```python
from build123d import *

# Parameters (mm, degrees)
ESQUISSE1_R             = 6
ESQUISSE1_R_2           = 1.6
EXTRUSION1_DEPTH        = 5
ESQUISSE2_W             = 10
ESQUISSE2_H             = 6
ENL_V_MAT_EXTRU_1_DEPTH = 2.5
ESQUISSE3_R             = 1.5
ENL_V_MAT_EXTRU_2_DEPTH = 28.658633372


with BuildPart() as part:
    # Esquisse1 → Extrusion1 (new body)
    with BuildSketch(Plane.XY):
        Polygon((-7, 16), (10, 16), (10, -16), (-7, -16), (-7, -7.5), (-12, -7.5), (-12, 7.5), (-7, 7.5), align=None)
        Circle(ESQUISSE1_R, mode=Mode.SUBTRACT)
        with Locations((-9, 0)):
            Circle(ESQUISSE1_R_2, mode=Mode.SUBTRACT)
        with Locations((4.5, 7.794228634)):
            Circle(ESQUISSE1_R_2, mode=Mode.SUBTRACT)
        with Locations((4.5, -7.794228634)):
            Circle(ESQUISSE1_R_2, mode=Mode.SUBTRACT)
    extrude(amount=EXTRUSION1_DEPTH)

    # Esquisse2 → Enlèv. mat.-Extru.1 (cut)
    with BuildSketch(Plane(origin=(0, 0, 0), x_dir=(-1, 0, 0), z_dir=(0, 0, -1))):
        with Locations((-5, 0)):
            Rectangle(ESQUISSE2_W, ESQUISSE2_H)
    extrude(amount=-ENL_V_MAT_EXTRU_1_DEPTH, mode=Mode.SUBTRACT)

    # Esquisse3 → Enlèv. mat.-Extru.2 (cut, through all)
    with BuildSketch(Plane.ZY.offset(12)):
        with Locations((2.5, 13)):
            Circle(ESQUISSE3_R)
        with Locations((2.5, -13)):
            Circle(ESQUISSE3_R)
    extrude(amount=-ENL_V_MAT_EXTRU_2_DEPTH, mode=Mode.SUBTRACT)


solid = part.part
```
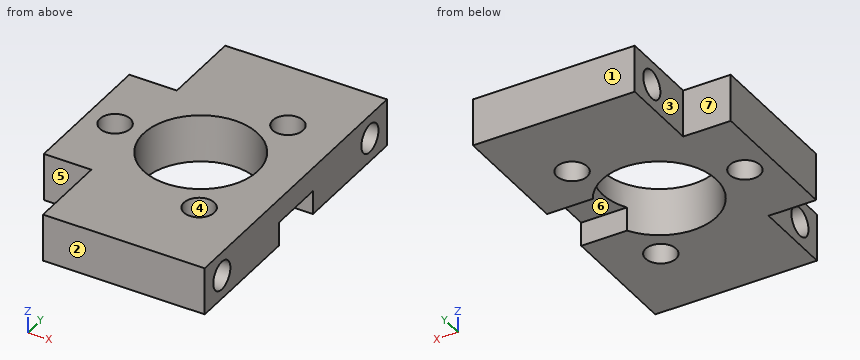
Geometry: final body of the model. Coordinates: model frame, mm. Face numbers are marked on the shaded views. A direction names the side the tool comes from. Give positions to 0.01 mm unless a question says otherwise; leave off trailing zeros. Write each loop counter-clockwise with the first axis right and the second up, starting at its lowest first coordinate (ties: lowest second). Pieces come first, ordered by that corner, then holes.
1. Section query A-A, the plane z = 3.55. Return loops of the section in (x, y), then the cut area to 3 significant figures.
2. Section query C-C, the plane x = -2. Return loops of the section in (y, z), then the cut area to 3 significant figures.
3. Section query B-B, the plane y = 13. Return loops of the section in (x, z).
4. Line query: probe 1 along Y at (x, z) = (-9, 2.95); probe 2 along Y at (x, z) = (4.5, 1.5); probe 3 along Y at (x, z) = (3.75, 2.5). Output: solid intervals per line, ascending.
5. Reachability of the marked faces 5, 6 and 7 from +Z, -Z, +X, -X, +Y, -Y: full face, straight path, thin tool, end or side. Return the list, or none.
6. Pin query (flat end, axial travel): P1, Ø1.5, axis at y = 11.5, z = 2, coming from the -X side; P2, Ø3, axis at x = 4.5, y = -7.79, coming from the +Z side; P3, Ø1, axis at x = -8.5, z = 2, coming from the -Y side; P4, Ø2.5, axis at x = -9.5, z = 2, coming from the +Y side. Return the tip coordinate at first contact, or that it passes through.
7. Section query D-D, the plane x = 3.25. Return loops of the section in (y, z), then the cut area to 3 significant figures.
8. Draft query along Y for the marked faces 1, 2, 3 and 4. Return one class per face: released by +Y, released by -Y, zero draft, split by the parting line, or undercut.
Computed:
1. outline: (-12, -7.5) - (-7, -7.5) - (-7, -11.93) - (10, -11.93) - (10, 11.93) - (-7, 11.93) - (-7, 7.5) - (-12, 7.5) - close; (-7, -16) - (10, -16) - (10, -14.07) - (-7, -14.07) - close; (-7, 14.07) - (10, 14.07) - (10, 16) - (-7, 16) - close; hole circle Ø3.2 at (-9, 0); hole circle Ø12 at (0, 0); hole circle Ø3.2 at (4.5, -7.79); hole circle Ø3.2 at (4.5, 7.79)
1. area: 409 mm2
2. outline: (-16, 0) - (-5.66, 0) - (-5.66, 5) - (-16, 5) - close; (5.66, 0) - (16, 0) - (16, 5) - (5.66, 5) - close; hole circle Ø3 at (-13, 2.5); hole circle Ø3 at (13, 2.5)
2. area: 89.3 mm2
3. outline: (-7, 0) - (10, 0) - (10, 1) - (-7, 1) - close; (-7, 4) - (10, 4) - (10, 5) - (-7, 5) - close
4. probe 1: y = -7.5 to -1.6, 1.6 to 7.5
4. probe 2: y = -16 to -14.12, -11.88 to -9.39, -6.19 to -3.97, 3.97 to 6.19, 9.39 to 11.88, 14.12 to 16
4. probe 3: y = -16 to -14.5, -11.5 to -9.21, -6.38 to -4.68, 4.68 to 6.38, 9.21 to 11.5, 14.5 to 16
5. face 5: +Z, -Z, -X, -Y
5. face 6: -Z, +X
5. face 7: +Z, -Z, -X, +Y
6. P1: stops at x = -7
6. P2: passes through
6. P3: stops at y = -7.5
6. P4: stops at y = 7.5
7. outline: (-16, 0) - (-8.79, 0) - (-8.79, 5) - (-16, 5) - close; (-6.8, 0) - (-5.04, 0) - (-5.04, 5) - (-6.8, 5) - close; (5.04, 0) - (6.8, 0) - (6.8, 5) - (5.04, 5) - close; (8.79, 0) - (16, 0) - (16, 5) - (8.79, 5) - close; hole circle Ø3 at (-13, 2.5); hole circle Ø3 at (13, 2.5)
7. area: 75.5 mm2
8. face 1: released by +Y
8. face 2: released by -Y
8. face 3: zero draft
8. face 4: undercut
